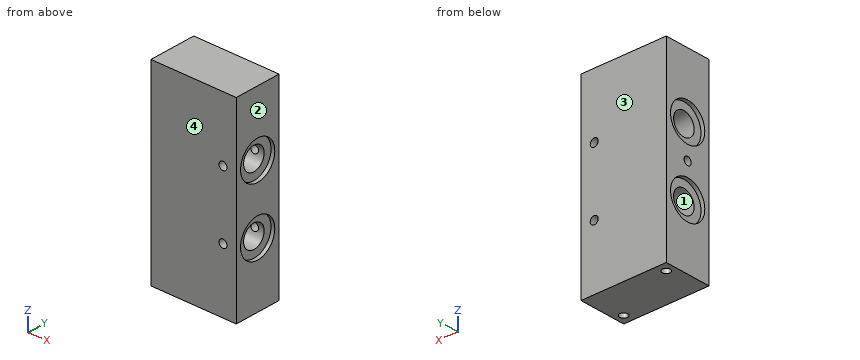
from build123d import *

# Parameters (mm, degrees)
SKETCH1_W             = 45
SKETCH1_H             = 102
BOSS_EXTRUDE1_DEPTH   = 25
M5_TAPPED_HOLE3_D     = 4.2
SKETCH27_R            = 6
CUT_EXTRUDE1_DEPTH    = 74
SKETCH28_R            = 10
CUT_EXTRUDE3_DEPTH    = 2
SKETCH30_R            = 10
CUT_EXTRUDE4_DEPTH    = 2
M5_TAPPED_HOLE4_D     = 4.2
M5_TAPPED_HOLE4_DEPTH = 14
M5_TAPPED_HOLE4_TIP   = 1.2618073
M5_TAPPED_HOLE5_D     = 4.2
M5_TAPPED_HOLE5_DEPTH = 15
M5_TAPPED_HOLE5_TIP   = 1.2618073


with BuildPart() as part:
    # Sketch1 → Boss-Extrude1 (new body)
    with BuildSketch(Plane(origin=(0, 0, 0), x_dir=(1, 0, 0), z_dir=(0, 1, 0))):
        Rectangle(SKETCH1_W, SKETCH1_H)
    extrude(amount=BOSS_EXTRUDE1_DEPTH)

    # M5 Tapped Hole3 (through all)
    with Locations(Plane(origin=(0, 25, 0), x_dir=(1, 0, 0), z_dir=(0, 1, 0))):
        with Locations((15.5, 17.5), (15.5, -17.5)):
            Hole(M5_TAPPED_HOLE3_D / 2)

    # Sketch27 → Cut-Extrude1 (cut)
    with BuildSketch(Plane.ZY.offset(22.5)):
        with Locations((-17.5, 12.5)):
            Circle(SKETCH27_R)
        with Locations((17.5, 12.5)):
            Circle(SKETCH27_R)
    extrude(amount=-CUT_EXTRUDE1_DEPTH, mode=Mode.SUBTRACT)

    # Sketch28 → Cut-Extrude3 (cut)
    with BuildSketch(Plane.ZY.offset(22.5)):
        with Locations((-17.5, 12.5)):
            Circle(SKETCH28_R)
        with Locations((17.5, 12.5)):
            Circle(SKETCH28_R)
    extrude(amount=-CUT_EXTRUDE3_DEPTH, mode=Mode.SUBTRACT)

    # Sketch30 → Cut-Extrude4 (cut)
    with BuildSketch(Plane(origin=(22.5, 0, 0), x_dir=(0, 0, -1), z_dir=(1, 0, 0))):
        with Locations((-17.5, 12.5)):
            Circle(SKETCH30_R)
        with Locations((17.5, 12.5)):
            Circle(SKETCH30_R)
    extrude(amount=-CUT_EXTRUDE4_DEPTH, mode=Mode.SUBTRACT)

    # M5 Tapped Hole4
    with Locations(Plane(origin=(0, 0, -51), x_dir=(-1, 0, 0), z_dir=(0, 0, -1))):
        with Locations((-18, 5), (18, 20)):
            Hole(M5_TAPPED_HOLE4_D / 2, depth=M5_TAPPED_HOLE4_DEPTH)
            with Locations((0, 0, -(M5_TAPPED_HOLE4_DEPTH + M5_TAPPED_HOLE4_TIP / 2))):  # 118° drill point
                Cone(0, M5_TAPPED_HOLE4_D / 2, M5_TAPPED_HOLE4_TIP, mode=Mode.SUBTRACT)

    # M5 Tapped Hole5
    with Locations(Plane.ZY.offset(22.5)):
        with Locations((0, 12.5)):
            Hole(M5_TAPPED_HOLE5_D / 2, depth=M5_TAPPED_HOLE5_DEPTH)
            with Locations((0, 0, -(M5_TAPPED_HOLE5_DEPTH + M5_TAPPED_HOLE5_TIP / 2))):  # 118° drill point
                Cone(0, M5_TAPPED_HOLE5_D / 2, M5_TAPPED_HOLE5_TIP, mode=Mode.SUBTRACT)


solid = part.part
Model file for the job. Use its own axes, mm. Face numbers are marked on the shaded views. Give positions to 0.01 mm unless a question says otherwise; leave off trailing zeros. Order: outer loops, then holes, each group sorted by start corner. A loop starts at its lowest first (then second) coordinate and runs counter-clockwise, first axis right, second up. Notation, with made-up numbers: (-25, 54) - (20, 54) arc R9 ccw to (20, 65) - close; hole circle Ø8 at (59.5, -23). An arc over 180 degrees is marked (long way). Write item = value, one per line. Start each with the question number.
1. Two-plate mould, pull along Y, no slides. Class the marked faces 1, 2, 3 and 4: pulls with the +Y half, pulls with the -Y half, needs draft (parallel to the pull), parting line crosses it, or undercut.
2. Cut at B-B, the plane x = 5. List the corners of the cut face in (y, z), and give its area (3 significant figures).
3. Cut at A-A, the plane z = -17.5. List the corners of the cut face in (x, y), and give its area (3 significant figures).
4. Probe line 1 along Y through (x, z) = (-18, -45.5); line 2 along Z through (x, y) = (15.5, 20); line 3 along Z through (x, y) = (-14, 15.5). List the from-to ranges inside material, lowest first.
5. Drop flat-ended pins along their axis: P1, Ø6.5, axis at x = -18, y = 20, coming from the -Z side; P2, Ø2.5, axis at x = 15.5, z = 17.5, coming from the -Y side; P3, Ø4, axis at y = 12.5, z = 0, coming from the -X side. Give the stop position or say it passes through.
Taken from the geometry:
q1.face_1 = undercut
q1.face_2 = needs draft
q1.face_3 = pulls with the +Y half
q1.face_4 = pulls with the -Y half
q2.outline = (0, -51) - (25, -51) - (25, 51) - (0, 51) - close; hole circle Ø12 at (12.5, -17.5); hole circle Ø12 at (12.5, 17.5)
q2.area = 2,320 mm²
q3.outline = (-22.5, 0) - (13.4, 0) - (13.4, 6.5) - (-20.5, 6.5) - (-20.5, 2.5) - (-22.5, 2.5) - close; (-22.5, 22.5) - (-20.5, 22.5) - (-20.5, 18.5) - (13.4, 18.5) - (13.4, 25) - (-22.5, 25) - close; (17.6, 0) - (22.5, 0) - (22.5, 2.5) - (20.5, 2.5) - (20.5, 6.5) - (17.6, 6.5) - close; (17.6, 18.5) - (20.5, 18.5) - (20.5, 22.5) - (22.5, 22.5) - (22.5, 25) - (17.6, 25) - close
q3.area = 498 mm²
q4.line_1 = 0 to 17.9, 22.1 to 25
q4.line_2 = -51 to -19.6, -15.4 to 15.4, 19.6 to 51
q4.line_3 = -51 to -22.7, -12.3 to 12.3, 22.7 to 51
q5.P1 = -51
q5.P2 = through
q5.P3 = -7.44
